Here's the drawing with two shaded views (mm, measured from the low corner). I have some questions. Give positions to 0.01 mm unless a question says otherwise; leave off trailing zeros. Write each loop counter-clockwise with the first axis right and the second up, starting at its lowest first coordinate (ties: lowest second). Pieces come first, ordered by that corner, then holes. Notation, with made-up numbers: (42.25, 46) -> (48.25, 46) arc R6 cw to (48.25, 51) -> close; hole circle Ø10 at (42, -6). An arc over 180 degrees is marked (long way). One line per item, written item: value.
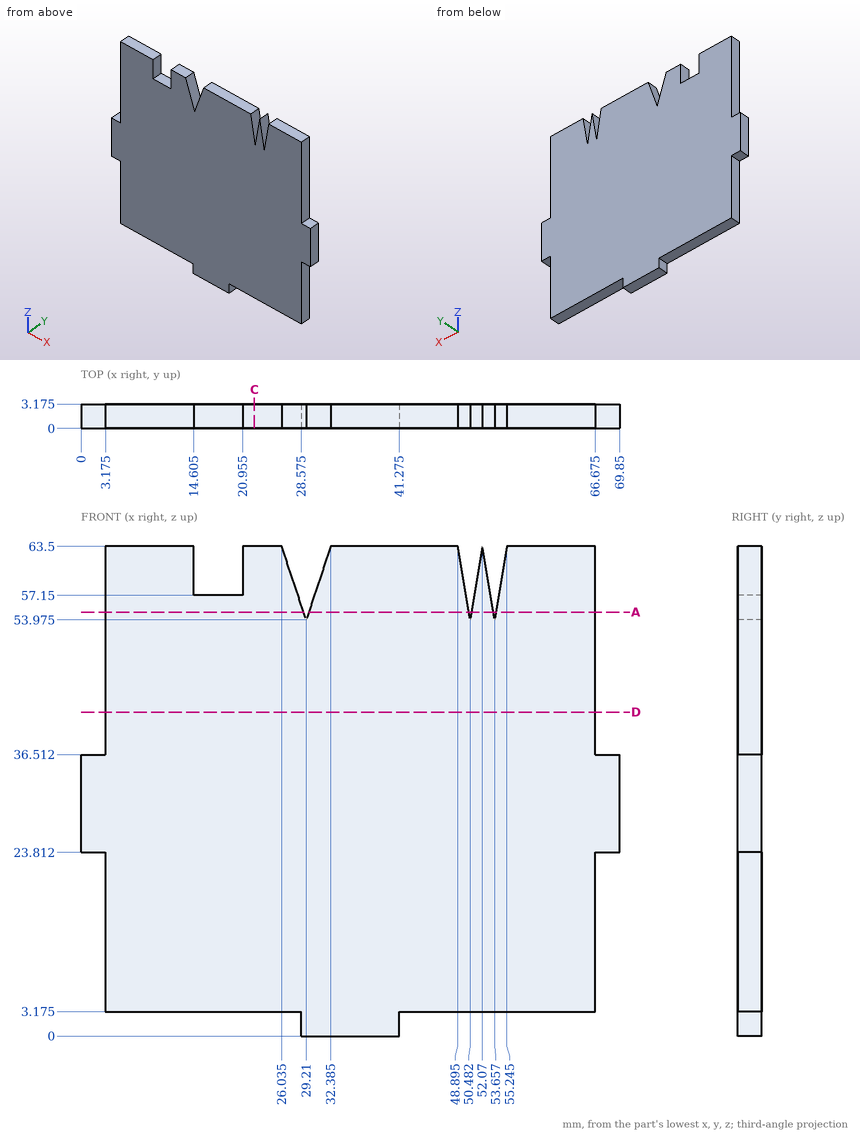
1) I need wall thicknesses on L1, parallel to X at y = 0.3, z = 17 (1 decimal); L2, parallel to Z at x = 61, y = 0.5 (1 decimal). Which ranges of each line are inside material? Lowest first, please.
Answer list:
L1: x = 3.2 to 66.7
L2: z = 3.2 to 63.5
2) Will these pins go through, and if not, where does the flat tip stop? pin 1 (1 mm diameter, centred on y = 1.5, z = 30, fed in from -X); pin 2 (1.6 mm diameter, centred on x = 48, y = 1, fed in from -Z) (1 decimal); pin 3 (1 mm diameter, centred on y = 1, z = 59, fed in from -X) (1 decimal); pin 4 (1 mm diameter, centred on x = 19, y = 1, fed in from +Z).
Answer list:
pin 1: stops at x = 0
pin 2: stops at z = 3.2
pin 3: stops at x = 3.2
pin 4: stops at z = 57.15
3) If we section it at C-C (x = 22.5): Write out the boundary of the cut face in (y, z) (1 decimal).
Answer list:
outline: (0, 3.2) -> (3.2, 3.2) -> (3.2, 63.5) -> (0, 63.5) -> close
4) If we section it at A-A (z = 55): Write out the boundary of the cut face in (x, y) (1 decimal).
Answer list:
outline: (3.2, 0) -> (28.9, 0) -> (28.9, 3.2) -> (3.2, 3.2) -> close; (29.6, 0) -> (50.3, 0) -> (50.3, 3.2) -> (29.6, 3.2) -> close; (50.7, 0) -> (53.5, 0) -> (53.5, 3.2) -> (50.7, 3.2) -> close; (53.8, 0) -> (66.7, 0) -> (66.7, 3.2) -> (53.8, 3.2) -> close
5) If we section it at D-D (z = 42): Write out the boundary of the cut face in (x, y) (1 decimal).
Answer list:
outline: (3.2, 0) -> (66.7, 0) -> (66.7, 3.2) -> (3.2, 3.2) -> close
